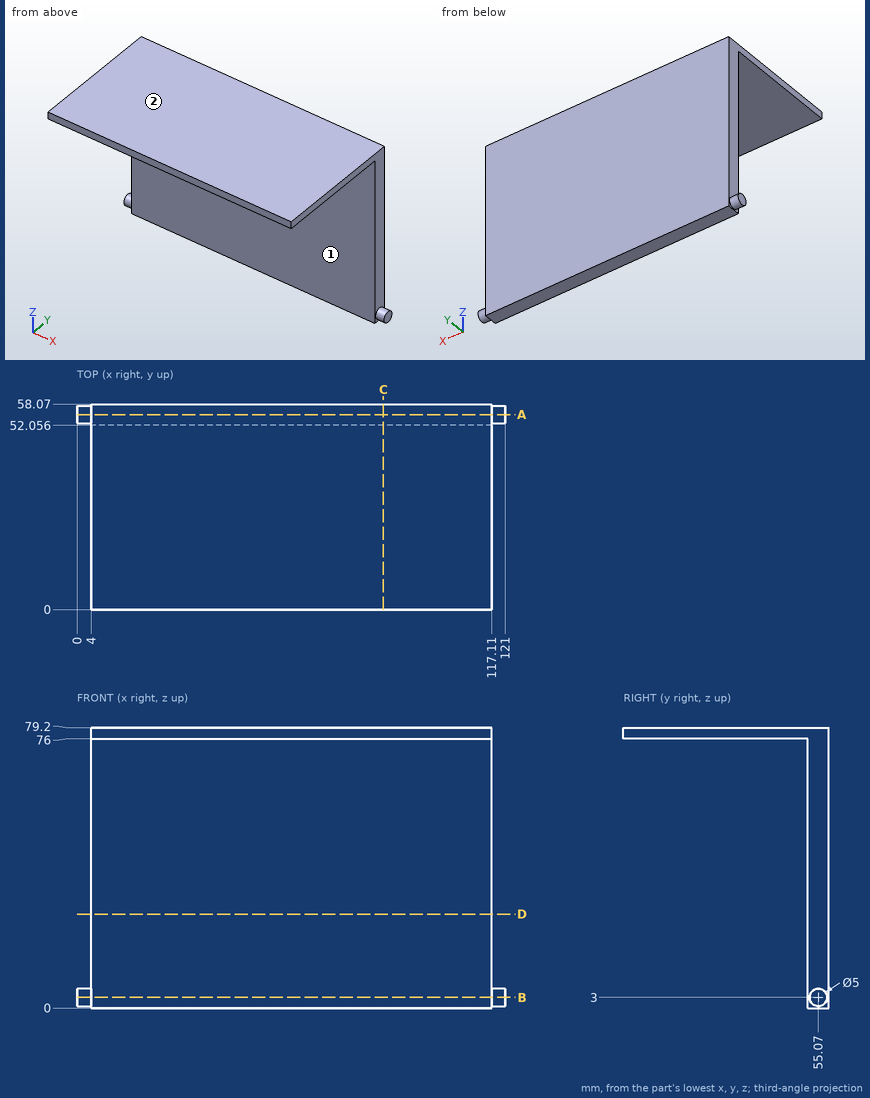
Answer from the drawing. Dimensions are ordinates in mm from the lowest x, y and z of the part. A direction names the side the tool comes from. Round coordinates to 2 decimals unless told otherwise and drop trailing zeros. Write each loop counter-clockwise with the first axis right and the second up, starting at its lowest first coordinate (ties: lowest second). Pieces come first, ordered by that corner, then holes. Notation, with made-up numbers: M -26.5,-19.5 L -7.5,-19.5 A11 cw -7.5,-5.5 Z; hole C 57.25,19.25 d4. An arc over 180 degrees is marked long. One line per item, written item: value.
Q1. Straight lines are drawn through the part: line 1 (Z direction, x = 94.5, y = 16); line 2 (Y direction, x = 57, z = 56) (1 decimal). For each, find the intervals that lie inside material, in ascending order. Write a range as [from, to].
Data:
line 1: [76, 79.2]
line 2: [52.1, 58.1]
Q2. Find section C-C on x = 86.5. Write down the section's boundary in (y, z) (1 decimal), plus the area to 3 significant figures.
Data:
outline: M 0,76 L 52.1,76 L 52.1,0 L 58.1,0 L 58.1,79.2 L 0,79.2 Z
area: 643 mm2
Q3. Find section B-B on z = 3. Write down the section's boundary in (x, y) (1 decimal), plus the area to 3 significant figures.
Data:
outline: M 0,52.6 L 4,52.6 L 4,52.1 L 117.1,52.1 L 117.1,52.6 L 121,52.6 L 121,57.6 L 117.1,57.6 L 117.1,58.1 L 4,58.1 L 4,57.6 L 0,57.6 Z
area: 720 mm2
Q4. Which of the six approach directions +Z, -Z, +X, -X, +Y, -Y give full straight-line access (tool end or side, diameter ignored) to the marked faces 1 and 2?
Data:
face 1: -Z, +X, -X, -Y
face 2: +Z, +X, -X, +Y, -Y
Q5. Flat-ended cylindrical pins translate along their axes: pin 1 Ø6 at (x, z) = (12.5, 28.5) entering from -Y; pin 2 Ø15.5 at (x, y) = (58, 24.5) entering from -Z. Find the tip coordinate at first contact, or state that the pin passes through.
Data:
pin 1: y = 52.06
pin 2: z = 76
Q6. Find section D-D on z = 26.5. Write down the section's boundary in (x, y) (1 decimal).
Data:
outline: M 4,52.1 L 117.1,52.1 L 117.1,58.1 L 4,58.1 Z
Q7. Find section A-A on y = 55.07. Write down the section's boundary in (x, z), plus the area to 3 significant figures.
Data:
outline: M 0,0.5 L 4,0.5 L 4,0 L 117.11,0 L 117.11,0.5 L 121,0.5 L 121,5.5 L 117.11,5.5 L 117.11,79.2 L 4,79.2 L 4,5.5 L 0,5.5 Z
area: 9,000 mm2
